```python
from build123d import *

# Parameters (mm, degrees)
SKETCH1_R           = 59.999999999
BOSS_EXTRUDE1_DEPTH = 50
SKETCH3_R           = 59.999999999
BOSS_EXTRUDE2_DEPTH = 10
FILLET1_R           = 10
FILLET2_R           = 10
SKETCH5_R           = 2.25
CUT_EXTRUDE2_DEPTH  = 6.1


with BuildPart() as part:
    # Sketch1 → Boss-Extrude1 (new body)
    with BuildSketch(Plane(origin=(0, 0, 0), x_dir=(1, 0, 0), z_dir=(0, 1, 0))):
        with Locations(Location((-1.875, 3e-09, 0), (0, 0, 270))):
            Circle(SKETCH1_R)
        with BuildLine():
            ThreePointArc((-50.028343877, 13.463115287), (-50.914264017, 9.754516103), (-51.514999998, 5.989190263))
            ThreePointArc((-51.514999998, 5.989190263), (-57.874999995, 3e-09), (-51.514999998, -5.989190257))
            ThreePointArc((-51.514999998, -5.989190257), (-50.914264017, -9.754516098), (-50.028343877, -13.463115281))
            ThreePointArc((-50.028343877, -13.463115281), (-53.612253816, -21.430272208), (-45.444416106, -24.529695876))
            ThreePointArc((-45.444416106, -24.529695876), (-43.448480613, -27.778511647), (-41.210777663, -30.865783567))
            ThreePointArc((-41.210777663, -30.865783567), (-41.472979743, -39.59797974), (-32.74078357, -39.33577766))
            ThreePointArc((-32.74078357, -39.33577766), (-29.653511649, -41.57348061), (-26.404695879, -43.569416103))
            ThreePointArc((-26.404695879, -43.569416103), (-23.30527221, -51.737253813), (-15.338115284, -48.153343875))
            ThreePointArc((-15.338115284, -48.153343875), (-11.6295161, -49.039264015), (-7.86419026, -49.639999995))
            ThreePointArc((-7.86419026, -49.639999995), (-1.875, -55.999999992), (4.11419026, -49.639999995))
            ThreePointArc((4.11419026, -49.639999995), (7.8795161, -49.039264015), (11.588115284, -48.153343875))
            ThreePointArc((11.588115284, -48.153343875), (19.55527221, -51.737253813), (22.654695879, -43.569416103))
            ThreePointArc((22.654695879, -43.569416103), (25.903511649, -41.57348061), (28.99078357, -39.33577766))
            ThreePointArc((28.99078357, -39.33577766), (37.722979743, -39.59797974), (37.460777663, -30.865783567))
            ThreePointArc((37.460777663, -30.865783567), (39.698480613, -27.778511647), (41.694416106, -24.529695876))
            ThreePointArc((41.694416106, -24.529695876), (49.862253816, -21.430272208), (46.278343877, -13.463115281))
            ThreePointArc((46.278343877, -13.463115281), (47.164264017, -9.754516098), (47.764999998, -5.989190257))
            ThreePointArc((47.764999998, -5.989190257), (54.124999995, 3e-09), (47.764999998, 5.989190263))
            ThreePointArc((47.764999998, 5.989190263), (47.164264017, 9.754516103), (46.278343877, 13.463115287))
            ThreePointArc((46.278343877, 13.463115287), (49.862253816, 21.430272213), (41.694416106, 24.529695882))
            ThreePointArc((41.694416106, 24.529695882), (39.698480613, 27.778511652), (37.460777663, 30.865783572))
            ThreePointArc((37.460777663, 30.865783572), (37.722979743, 39.597979745), (28.99078357, 39.335777666))
            ThreePointArc((28.99078357, 39.335777666), (25.903511649, 41.573480616), (22.654695879, 43.569416109))
            ThreePointArc((22.654695879, 43.569416109), (19.55527221, 51.737253819), (11.588115284, 48.15334388))
            ThreePointArc((11.588115284, 48.15334388), (7.8795161, 49.03926402), (4.11419026, 49.64))
            ThreePointArc((4.11419026, 49.64), (-1.875, 55.999999998), (-7.86419026, 49.64))
            ThreePointArc((-7.86419026, 49.64), (-11.6295161, 49.03926402), (-15.338115284, 48.15334388))
            ThreePointArc((-15.338115284, 48.15334388), (-23.30527221, 51.737253819), (-26.404695879, 43.569416109))
            ThreePointArc((-26.404695879, 43.569416109), (-29.653511649, 41.573480616), (-32.74078357, 39.335777666))
            ThreePointArc((-32.74078357, 39.335777666), (-41.472979743, 39.597979745), (-41.210777663, 30.865783572))
            ThreePointArc((-41.210777663, 30.865783572), (-43.448480613, 27.778511652), (-45.444416106, 24.529695882))
            ThreePointArc((-45.444416106, 24.529695882), (-53.612253816, 21.430272213), (-50.028343877, 13.463115287))
        make_face(mode=Mode.SUBTRACT)
    extrude(amount=BOSS_EXTRUDE1_DEPTH)

    # Sketch3 → Boss-Extrude2 (add)
    with BuildSketch(Plane(origin=(0, 0, 0), x_dir=(1, 0, 0), z_dir=(0, 1, 0))):
        with Locations(Location((-1.875, 3e-09, 0), (0, 0, 270))):
            Circle(SKETCH3_R)
    extrude(amount=BOSS_EXTRUDE2_DEPTH)

    # Fillet1
    # the kernel refuses this fillet: 10 mm, written as the material it takes off along each edge
    with BuildSketch(Plane(origin=(11.588115284, 10, -48.15334388), x_dir=(-0.9762460203923251, 0, -0.2166649664070039), z_dir=(0, 1, 0))) as fillet1_piece_1:
        with BuildLine():
            CenterArc((5.962374186, -9.98529915), FILLET1_R, 93.107148893, 45.06938167)
            ThreePointArc((-1.489654942, -3.316921396), (-0.487517252, -1.774020699), (0, 0))
            ThreePointArc((0, 0), (2.710170085, -0.073504248), (5.420340169, 0))
        make_face()
    extrude(amount=53.550850423, mode=Mode.SUBTRACT)
    with BuildSketch(Plane(origin=(4.11419026, 10, -49.64), x_dir=(0.9848478099539646, 0, 0.17342085004081753), z_dir=(0, 1, 0))) as fillet1_piece_2:
        with BuildLine():
            CenterArc((5.962374186, 9.98529915), FILLET1_R, 221.823469437, 45.06938167)
            ThreePointArc((-1.489654942, 3.316921396), (-0.487517252, 1.774020699), (0, 0))
            ThreePointArc((0, 0), (2.710170085, 0.073504248), (5.420340169, 0))
        make_face()
    extrude(amount=53.550850423, mode=Mode.SUBTRACT)

    # Fillet2
    # the kernel refuses this fillet: 10 mm, written as the material it takes off along each edge
    with BuildSketch(Plane(origin=(-50.028343877, 10, -13.463115287), x_dir=(-0.8017919038554878, 0, -0.5976033324135602), z_dir=(0, 1, 0)), Plane(origin=(-51.514999998, 10, 5.989190257), x_dir=(-0.9694520237461802, 0, -0.24528100956746685), z_dir=(0, 1, 0)), Plane(origin=(-45.444416106, 10, 24.529695876), x_dir=(-0.9895218611259949, 0, 0.14438312350737928), z_dir=(0, 1, 0)), Plane(origin=(-32.74078357, 10, 39.33577766), x_dir=(-0.8589459651873854, 0, 0.5120662348645055), z_dir=(0, 1, 0)), Plane(origin=(-15.338115284, 10, 48.153343875), x_dir=(-0.5976033324135606, 0, 0.8017919038554876), z_dir=(0, 1, 0)), Plane(origin=(-41.210777663, 10, -30.865783572), x_dir=(-0.512066234864506, 0, -0.8589459651873851), z_dir=(0, 1, 0)), Plane(origin=(-26.404695879, 10, -43.569416109), x_dir=(-0.14438312350738092, 0, -0.9895218611259947), z_dir=(0, 1, 0)), Plane(origin=(-7.86419026, 10, -49.64), x_dir=(0.2452810095674737, 0, -0.9694520237461783), z_dir=(0, 1, 0)), Plane(origin=(4.11419026, 10, 49.639999995), x_dir=(-0.24528100956747004, 0, 0.9694520237461793), z_dir=(0, 1, 0)), Plane(origin=(22.654695879, 10, 43.569416103), x_dir=(0.14438312350738092, 0, 0.9895218611259947), z_dir=(0, 1, 0)), Plane(origin=(37.460777663, 10, 30.865783567), x_dir=(0.5120662348645055, 0, 0.8589459651873854), z_dir=(0, 1, 0)), Plane(origin=(46.278343877, 10, 13.463115281), x_dir=(0.8017919038554872, 0, 0.5976033324135612), z_dir=(0, 1, 0)), Plane(origin=(47.764999998, 10, -5.989190263), x_dir=(0.9694520237461796, 0, 0.24528100956746887), z_dir=(0, 1, 0)), Plane(origin=(41.694416106, 10, -24.529695882), x_dir=(0.9895218611259945, 0, -0.14438312350738228), z_dir=(0, 1, 0)), Plane(origin=(28.99078357, 10, -39.335777666), x_dir=(0.8589459651873865, 0, -0.5120662348645036), z_dir=(0, 1, 0))) as fillet2_piece_1:
        with BuildLine():
            CenterArc((6.666136994, 9.529885762), FILLET2_R, 207.292364441, 45.06938167)
            ThreePointArc((-2.220646476, 4.944574479), (-1.043270762, 2.502401023), (0, 0))
            ThreePointArc((0, 0), (1.818037362, 0.282068543), (3.636074723, 0))
        make_face()
    extrude(amount=53.550850423, mode=Mode.SUBTRACT)
    with BuildSketch(Plane(origin=(-51.514999998, 10, -5.989190263), x_dir=(0.17342085004081384, 0, -0.9848478099539651), z_dir=(0, 1, 0)), Plane(origin=(-50.028343877, 10, 13.463115281), x_dir=(-0.21666496640700172, 0, -0.9762460203923256), z_dir=(0, 1, 0)), Plane(origin=(-41.210777663, 10, 30.865783567), x_dir=(-0.5737655057921729, 0, -0.8190196239181647), z_dir=(0, 1, 0)), Plane(origin=(-26.404695879, 10, 43.569416103), x_dir=(-0.8435154481177425, 0, -0.5371049141338442), z_dir=(0, 1, 0)), Plane(origin=(-7.86419026, 10, 49.639999995), x_dir=(-0.9848478099539649, 0, -0.17342085004081545), z_dir=(0, 1, 0)), Plane(origin=(-45.444416106, 10, -24.529695882), x_dir=(0.537104914133847, 0, -0.8435154481177406), z_dir=(0, 1, 0)), Plane(origin=(-32.74078357, 10, -39.335777666), x_dir=(0.8190196239181653, 0, -0.5737655057921723), z_dir=(0, 1, 0)), Plane(origin=(-15.338115284, 10, -48.15334388), x_dir=(0.9762460203923244, 0, -0.21666496640700658), z_dir=(0, 1, 0)), Plane(origin=(11.588115284, 10, 48.153343875), x_dir=(-0.9762460203923242, 0, 0.2166649664070072), z_dir=(0, 1, 0)), Plane(origin=(28.99078357, 10, 39.33577766), x_dir=(-0.8190196239181662, 0, 0.5737655057921711), z_dir=(0, 1, 0)), Plane(origin=(41.694416106, 10, 24.529695876), x_dir=(-0.5371049141338422, 0, 0.8435154481177437), z_dir=(0, 1, 0)), Plane(origin=(47.764999998, 10, 5.989190257), x_dir=(-0.17342085004081517, 0, 0.984847809953965), z_dir=(0, 1, 0)), Plane(origin=(46.278343877, 10, -13.463115287), x_dir=(0.21666496640700275, 0, 0.9762460203923252), z_dir=(0, 1, 0)), Plane(origin=(37.460777663, 10, -30.865783572), x_dir=(0.5737655057921707, 0, 0.8190196239181664), z_dir=(0, 1, 0))) as fillet2_piece_2:
        with BuildLine():
            CenterArc((5.962374186, 9.98529915), FILLET2_R, 221.823469437, 45.06938167)
            ThreePointArc((-1.489654942, 3.316921396), (-0.487517252, 1.774020699), (0, 0))
            ThreePointArc((0, 0), (2.710170085, 0.073504248), (5.420340169, 0))
        make_face()
    extrude(amount=53.550850423, mode=Mode.SUBTRACT)
    with BuildSketch(Plane(origin=(22.654695879, 10, -43.569416109), x_dir=(0.14438312350738122, 0, -0.9895218611259947), z_dir=(0, 1, 0))) as fillet2_piece_3:
        with BuildLine():
            CenterArc((6.666136994, -9.529885762), FILLET2_R, 107.638253889, 45.06938167)
            ThreePointArc((-2.220646476, -4.944574479), (-1.043270762, -2.502401023), (0, 0))
            ThreePointArc((0, 0), (1.818037362, -0.282068543), (3.636074723, 0))
        make_face()
    extrude(amount=53.550850423, mode=Mode.SUBTRACT)

    # Sketch5 → Cut-Extrude2 (cut)
    with BuildSketch(Plane(origin=(0, 50, 0), x_dir=(1, 0, 0), z_dir=(0, 1, 0))):
        with Locations(Location((7.985878763, 54.108807696, 0), (0, 0, 270))):
            Circle(SKETCH5_R)
        with Locations(Location((-55.983807694, 9.860878766, 0), (0, 0, 270))):
            Circle(SKETCH5_R)
        with Locations(Location((-11.735878763, -54.108807691, 0), (0, 0, 270))):
            Circle(SKETCH5_R)
        with Locations(Location((52.233807694, -9.86087876, 0), (0, 0, 270))):
            Circle(SKETCH5_R)
    extrude(amount=-CUT_EXTRUDE2_DEPTH, mode=Mode.SUBTRACT)


solid = part.part
```
Design review of the part built by this model. Coordinates are the model's own, in mm. Coordinates: 2 decimals unless noted, no trailing zeros. Write each loop counter-clockwise with the first axis right and the second up, starting at its lowest first coordinate (ties: lowest second). Pieces come first, ordered by that corner, then holes.
1) Add section A-A (z = 0). Write out the cut boundary in (x, y) (3 decimals).
2) Mouldability with a two-part tool opening along Z and no side actions: class faces 1 (the flat face through (43, 50, 26)), 2 (the cylindrical face through (39.09, 29.72, -30.93)), 3 (the cylindrical face through (-60.448, 24.65, -13.007)) as +Z half, -Z half, draft (parallel to the pull), parting line (faces both ways), or undercut.
3) Add section B-B (x = 20.5). Write out the cut boundary in (y, z), plus the area to 3 significant figures.
4) Insertion check: pin 1 (3 mm diameter, centred on x = -6, y = 29.5, fed in from -Z); pin 2 (12 mm diameter, centred on y = 32.5, z = -24.5, fed in from -X); pin 3 (6 mm diameter, centred on x = -11.5, y = 40, fed in from +Z). Each pin has a flat end and moves straight along its axis. Give the tip position at first contact, or say it passes through.
5) To check wall thickness, follow L1, parallel to X at y = 44.5, z = -50.5; L2, parallel to Y at x = -51, z = -12; L3, parallel to Z at x = 9, y = 28. State the ranges of each line that lie inside material, in increasing order.
Check result:
1. outline: (-61.875, 0) - (58.125, 0) - (58.125, 50) - (54.125, 50) - (54.125, 10) - (-57.875, 10) - (-57.875, 50) - (-61.875, 50) - close
2. face 1: draft
2. face 2: undercut
2. face 3: parting line
3. outline: (0, -55.67) - (50, -55.67) - (50, -51.24) - (10, -51.24) - (10, 51.24) - (50, 51.24) - (50, 55.67) - (0, 55.67) - close
3. area: 1,470 mm2
4. pin 1: stops at z = -59.94
4. pin 2: stops at x = -58.95
4. pin 3: stops at z = 59.63
5. L1: x = -34.27 to -25.19, -16.62 to -9.39, 5.64 to 12.87, 21.44 to 30.52
5. L2: y = 0 to 10
5. L3: z = -59.01 to -49.25, 49.25 to 59.01
